Could you check a few things on this model? Use its own coordinates, in mm. A direction names the side the tool comes from. Give positions to 0.01 mm unless a question says otherwise; leave off trailing zeros. Loops run counter-clockwise (first coordinate to the right, second up) from the corner with the lowest first, then second, coordinate; pieces in that order, holes last. Notation, with made-up numbers: M 78.25,54.5 L 93.25,54.5 A23 ccw 93.25,74.5 Z; hole C -37,57.5 d2. An arc over 180 degrees is marked long. Write each question's results on one line, items separated by ' | '. Start each with the question number.
from build123d import *

# Parameters (mm, degrees)
CUT_EXTRUDE_1_DEPTH = 2


with BuildPart() as part:
    # 草图1 → 旋转1 (revolve)
    with BuildSketch(Plane(origin=(0, 0, 0), x_dir=(1, 0, 0), z_dir=(0, 1, 0)), mode=Mode.PRIVATE) as revolve_1_sk:
        Polygon((0, 0), (2, 0), (2, 10), (3.5, 10), (3.5, 14), (0, 14), align=None)
    revolve(revolve_1_sk.sketch.rotate(Axis((0, 0, -14), (0, 0, 1)), 180), axis=Axis((0, 0, -14), (0, 0, 1)))

    # 草图2 → 切除-拉伸1 (cut)
    with BuildSketch(Plane(origin=(0, 0, -14), x_dir=(-1, 0, 0), z_dir=(0, 0, -1))):
        Polygon((0, 2.193931023), (-1.9, 1.096965511), (-1.9, -1.096965511), (0, -2.193931023), (1.9, -1.096965511), (1.9, 1.096965511), align=None)
    extrude(amount=-CUT_EXTRUDE_1_DEPTH, mode=Mode.SUBTRACT)


solid = part.part
1) If we section it at C-C on z = -11.5: Write out the boundary of the cut face in (x, y), plus the area to 3 significant figures.
2) Which directions (+Z, -Z, +X, -X, +Y, -Y) give clear straight access to the entire face, cutting with the end or side of a thin tool? Please do faces 1 (the face through (0.96, -1.64, -13.01)), 2 (the face through (2, 2, -10)), 3 (the face through (-3.233, 1.341, -12.028)).
3) If we section it at A-A on y = 0: Write out the boundary of the cut face in (x, z), plus the area to 3 significant figures.
4) If we section it at B-B on x = 0.5: Write out the boundary of the cut face in (y, z).
5) If we section it at D-D on z = -3.5: Write out the boundary of the cut face in (x, y).
6) Thinking about a two-plate mould opening in Y: for faces 4 (the face through (0, 0, 0)), 5 (the face through (0, 2, -5)), 6 (the face through (0.94, 1.65, -13.01)), which applies, pulls with the +Y half, pulls with the -Y half, needs draft (parallel to the pull), parting line crosses it, or undercut?
7) Please list where these lines run through material, in increasing order: line 1 (Z direction, x = 2, y = -0.5); line 2 (Z direction, x = 0, y = 1.25); line 3 (X direction, y = 0.5, z = -2). Write a range as from..to.
8) I'm going to push flat-ended pins straight in: P1, Ø0.6, axis at y = -0.5, z = -13.5, coming from the -X side; P2, Ø3, axis at x = -1.5, z = -3.5, coming from the +Y side; P3, Ø1.5, axis at y = 2.5, z = -5, coming from the -X side. Where does each tip first touch, or does it pass through?
Calculated:
1) outline: C 0,0 d7 | area: 38.5 mm2
2) face 1: -Z | face 2: +Z | face 3: +Z, -Z
3) outline: M -3.5,-14 L -1.9,-14 L -1.9,-12 L 1.9,-12 L 1.9,-14 L 3.5,-14 L 3.5,-10 L 2,-10 L 2,0 L -2,0 L -2,-10 L -3.5,-10 Z | area: 60.4 mm2
4) outline: M -3.46,-14 L -1.91,-14 L -1.91,-12 L 1.91,-12 L 1.91,-14 L 3.46,-14 L 3.46,-10 L 1.94,-10 L 1.94,0 L -1.94,0 L -1.94,-10 L -3.46,-10 Z
5) outline: C 0,0 d4
6) face 4: needs draft | face 5: parting line crosses it | face 6: undercut
7) line 1: z = -14..-10 | line 2: z = -12..0 | line 3: x = -1.94..1.94
8) P1: stops at x = -3.49 | P2: stops at y = 2 | P3: stops at x = -0.97
